from build123d import *

# Parameters (mm, degrees)
SKETCH_1_W             = 110
SKETCH_1_H             = 8
EXTRUDE_1_DEPTH        = 164.55
SKETCH_7_W             = 28
SKETCH_7_H             = 15
EXTRUDE_2_DEPTH        = 45
FILLET_1_R             = 50
SKETCH_10_R            = 12.215
CUT_EXTRUDE_3_DEPTH    = 10
SKETCH_11_R            = 2.5
CUT_EXTRUDE_4_DEPTH    = 30
FILLET_1_OF_MIRROR_1_R = 50
SKETCH_13_W            = 28
SKETCH_13_H            = 10
EXTRUDE_3_DEPTH        = 35
FILLET_2_R             = 50
SKETCH_14_R            = 3.975
EXTRUDE_4_DEPTH        = 15
MIRROR_START           = -44.153846154
MIRROR_2_DEPTH         = 28
MIRROR_START_2         = 10
MIRROR_2_2_OUTLINE_R   = 3.975
MIRROR_2_2_DEPTH       = 15


with BuildPart() as part:
    # Эскиз1 → Бобышка-Вытянуть1 (new body)
    with BuildSketch(Plane.XY):
        with Locations((0.846153846, 10.153846154)):
            Rectangle(SKETCH_1_W, SKETCH_1_H)
    extrude(amount=EXTRUDE_1_DEPTH)

    # Эскиз7 → Бобышка-Вытянуть2 (add)
    with BuildSketch(Plane.XZ.offset(-6.153846154)):
        with Locations((31.846153846, 157.05)):
            Rectangle(SKETCH_7_W, SKETCH_7_H)
    extrude_2 = extrude(amount=EXTRUDE_2_DEPTH)

    # Скругление1
    # the kernel refuses this fillet: 50 mm, written as the material it takes off along each edge
    with BuildSketch(Plane(origin=(135.114009203, -38.846153846, 164.55), x_dir=(0, 1, 0), z_dir=(-1, 0, 0))) as fillet_1_piece_1:
        with BuildLine():
            CenterArc((35.707142143, 50), FILLET_1_R, 224.427004001, 45.572995999)
            Line((0, 15), (-0.714142843, 14.3))
            ThreePointArc((-0.714142843, 14.3), (-1, 7.5), (-1, 0))
            Line((-1, 0), (0, -1))
            Line((0, -1), (35.707142143, -1))
            Line((35.707142143, -1), (35.707142143, 0))
        make_face()
    extrude(amount=206.535710714, mode=Mode.SUBTRACT)

    # Эскиз10 → Вырез-Вытянуть3 (cut)
    with BuildSketch(Plane(origin=(0, 0, 149.55), x_dir=(-1, 0, 0), z_dir=(0, 0, -1))):
        with Locations((-31.846153846, -23.846153846)):
            Circle(SKETCH_10_R)
    cut_extrude_3 = extrude(amount=-CUT_EXTRUDE_3_DEPTH, mode=Mode.SUBTRACT)

    # Эскиз11 → Вырез-Вытянуть4 (cut)
    with BuildSketch(Plane(origin=(0, 14.153846154, 0), x_dir=(1, 0, 0), z_dir=(0, 1, 0))):
        with Locations(Location((31.846153846, -159.55, 0), (0, 0, 270))):
            Circle(SKETCH_11_R)
    cut_extrude_4 = extrude(amount=-CUT_EXTRUDE_4_DEPTH, mode=Mode.SUBTRACT)

    # Зеркальное отражение1: Бобышка-Вытянуть2, Вырез-Вытянуть3, Вырез-Вытянуть4 across plane
    add(extrude_2.mirror(Plane.ZY.offset(-0.846153846)))
    add(cut_extrude_3.mirror(Plane.ZY.offset(-0.846153846)), mode=Mode.SUBTRACT)
    add(cut_extrude_4.mirror(Plane.ZY.offset(-0.846153846)), mode=Mode.SUBTRACT)

    # Скругление1 of Зеркальное отражение1
    # the kernel refuses this fillet: 50 mm, written as the material it takes off along each edge
    with BuildSketch(Plane(origin=(-133.421701511, -38.846153846, 164.55), x_dir=(0, 1, 0), z_dir=(1, 0, 0))) as fillet_1_of_mirror_1_piece_1:
        with BuildLine():
            CenterArc((35.707142143, -50), FILLET_1_OF_MIRROR_1_R, 90, 45.572995999)
            Line((0, -15), (-0.714142843, -14.3))
            ThreePointArc((-0.714142843, -14.3), (-1, -7.5), (-1, 0))
            Line((-1, 0), (0, 1))
            Line((0, 1), (35.707142143, 1))
            Line((35.707142143, 1), (35.707142143, 0))
        make_face()
    extrude(amount=206.535710714, mode=Mode.SUBTRACT)

    # Эскиз13 → Бобышка-Вытянуть3 (add)
    with BuildSketch(Plane(origin=(0, 6.153846154, 0), x_dir=(-1, 0, 0), z_dir=(0, -1, 0))):
        with Locations((-31.846153846, -5)):
            Rectangle(SKETCH_13_W, SKETCH_13_H)
    extrude(amount=EXTRUDE_3_DEPTH)

    # Скругление2
    # the kernel refuses this fillet: 50 mm, written as the material it takes off along each edge
    with BuildSketch(Plane(origin=(-57.153846154, -28.846153846, 0), x_dir=(0, 1, 0), z_dir=(1, 0, 0))) as fillet_2_piece_1:
        with BuildLine():
            CenterArc((30, 50), FILLET_2_R, 233.130102354, 36.869897646)
            Line((0, 10), (0, 0))
            Line((0, 0), (30, 0))
        make_face()
    extrude(amount=178, mode=Mode.SUBTRACT)

    # Эскиз14 → Бобышка-Вытянуть4 (add)
    with BuildSketch(Plane.XY.offset(10)):
        with Locations(Location((30.846153846, -23.846153846, 0), (0, 0, 180))):
            Circle(SKETCH_14_R)
    extrude(amount=EXTRUDE_4_DEPTH)

    # Зеркальное отражение2: read off the stored shape, not the designer's step
    # Зеркальное отражение2 outline → Зеркальное отражение2 (add)
    with BuildSketch(Plane.YZ.offset(MIRROR_START)):
        with BuildLine():
            Line((1.153846154, 0), (6.153846154, 0))
            Line((6.153846154, 0), (6.153846154, 10))
            Line((6.153846154, 10), (-28.846153846, 10))
            ThreePointArc((-28.846153846, 10), (-14.657542147, 2.565835097), (1.153846154, 0))
        make_face()
    extrude(amount=MIRROR_2_DEPTH)

    # Mirror 2 2 outline → Mirror 2 2 (add)
    with BuildSketch(Plane.XY.offset(MIRROR_START_2)):
        with Locations((-29.153846154, -23.846153846)):
            Circle(MIRROR_2_2_OUTLINE_R)
    extrude(amount=MIRROR_2_2_DEPTH)


solid = part.part
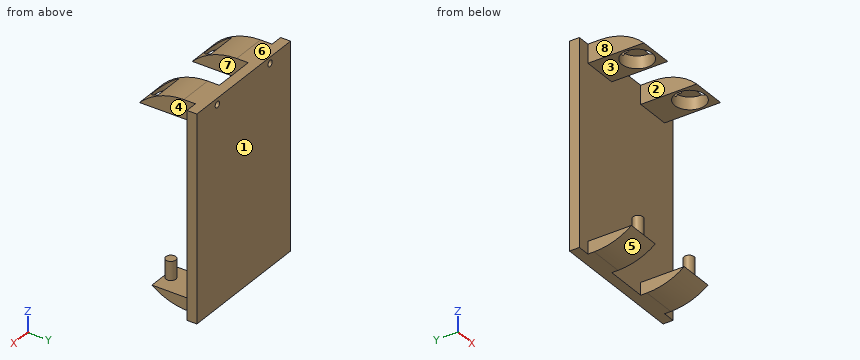
Check sheet for the modelled part. Datum: model origin and axes. Units: mm. Face numbers are marked on the shaded views. A direction names the side the tool comes from. Give positions to 0.01 mm unless a question says otherwise; leave off trailing zeros. Write each loop counter-clockwise with the first axis right and the second up, starting at its lowest first coordinate (ties: lowest second). Pieces come first, ordered by that corner, then holes. Notation, with made-up numbers: M 68,59.25 L 100,59.25 A15 cw 100,87.25 Z; hole C 33,5.25 d5. An arc over 180 degrees is marked long. Use one line per item in the form item = value.
(1) Depth check by flat-ended pin: P1, Ø1.5, axis at x = 42.5, y = -5, coming from the +Z side; P2, Ø8, axis at y = -3, z = 3, coming from the -X side; P3, Ø4, axis at x = -32, y = -25.5, coming from the +Z side; P4, Ø1, axis at x = -15.5, y = -11, coming from the -Z side. Enter the tip coordinate at first touch or a pass-through.
Answer block:
P1 = 164.54
P2 = -44.15
P3 = 160.22
P4 = through
(2) Section check A-A on y = -9.5. Record the boundary of the cut face in (x, z).
Answer block:
outline = M -44.15,1.15 L -16.15,1.15 L -16.15,10 L -44.15,10 Z; M -44.15,149.55 L -16.15,149.55 L -16.15,164.14 L -44.15,164.14 Z; M 17.85,1.15 L 45.85,1.15 L 45.85,10 L 17.85,10 Z; M 17.85,149.55 L 45.85,149.55 L 45.85,164.14 L 17.85,164.14 Z; hole C -30.15,159.55 d5; hole C 31.85,159.55 d5
(3) Draft check along X on the marked faces 6, 7 and 8. Enter one of: pulls with the +X half, pulls with the -X half, needs draft (parallel to the pull), parting line crosses it, or undercut.
Answer block:
face_6 = needs draft
face_7 = undercut
face_8 = pulls with the -X half
(4) Section check C-C on z = 92. Record the boundary of the cut face in (x, y).
Answer block:
outline = M -54.15,6.15 L 55.85,6.15 L 55.85,14.15 L -54.15,14.15 Z
(5) Section check B-B on x = -11. Record the boundary of the cut face in (y, z).
Answer block:
outline = M 6.15,0 L 14.15,0 L 14.15,164.55 L 6.15,164.55 Z
(6) Material ranges on line 1 along Z through (x, y) = (-36.5, 1); line 2 along Y through (x, z) = (-34, 45); line 3 along Z through (x, y) = (-35, -16), recorded low to high.
Answer block:
line_1 = 0 to 10, 149.55 to 164.55
line_2 = 6.15 to 14.15
line_3 = 3.03 to 10, 159.55 to 162.87
(7) Tool access check on the marked faces 1, 2, 3, 4 and 5. Record the directions out of +Z, -Z, +X, -X, +Y, -Y that give a thin tool (end or side, any length) a straight path to the whole face; none if there is none.
Answer block:
face_1 = +Z, -Z, +X, -X, +Y
face_2 = +Z, -Z, -Y
face_3 = +X, -X, -Y
face_4 = +Z, -Z, +X, -Y
face_5 = -Z, +X, -X, -Y
